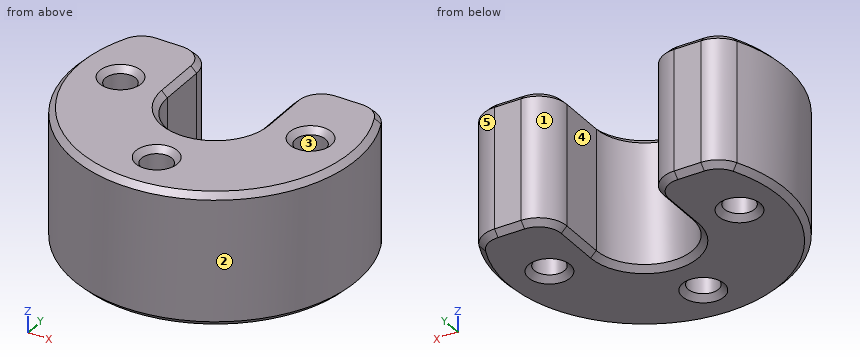
Autodesk Inventor part; units mm, degrees
ref_plane "YZ Plane" through (0, 0, 0) normal (1, 0, 0) x (0, 1, 0)
ref_plane "XZ Plane" through (0, 0, 0) normal (0, 1, 0) x (-1, 0, 0)
ref_plane "XY Plane" through (0, 0, 0) normal (0, 0, 1) x (1, 0, 0)
sketch "Эскиз1" plane through (0, 0, 0) normal (0, 0, 1) x (1, 0, 0)
  circle A0 centre (0, 0) radius 5.1
  circle A1 centre (0, 0) radius 15
  line L0 (0, -21) -> (0, 21) construction
  line L1 (-21, 0) -> (21, 0) construction
  circle A2 centre (0, 0) radius 10.05 construction
  circle A3 centre (-10.05, 0) radius 1.6
  circle A4 centre (0, -10.05) radius 1.6
  circle A5 centre (10.05, 0) radius 1.6
  line L2 (-12.6886, 8) -> (12.6886, 8)
  line L3 (-5.1, 0) -> (-5.1, 8)
  line L4 (5.1, 0) -> (5.1, 8)
  dimension "d0" = 10.2
  dimension "d1" = 30
  dimension "d2" = 20.1
  dimension "d3" = 3.2
  dimension "d4" = 8
extrude "Выдавливание1" add sketch "Эскиз1" along normal blind 14 contours L4 L2 A1 L3 A0
fillet "Сопряжение1" radius 3 4 edges at (-12.6886, 8, 7) (-5.1, 8, 7) (5.1, 8, 7) (12.6886, 8, 7)
chamfer "Фаска1" distance 0.6 angle 45 26 edges at (-5.9787, 7.1213, 14) (-5.1, 2.5, 14) (0, -5.1, 14) (5.1, 2.5, 14) (5.9787, 7.1213, 14) (9.5044, 8, 14) (12.5289, 7.5249, 14) (0, -15, 14) (-12.5289, 7.5249, 14) (-9.5044, 8, 14) (-11.65, 0, 14) (-1.6, -10.05, 14) (8.45, 0, 14) (0, -5.1, 0) (-5.1, 2.5, 0) (-5.9787, 7.1213, 0) (-9.5044, 8, 0) (-12.5289, 7.5249, 0) (0, -15, 0) (12.5289, 7.5249, 0) (9.5044, 8, 0) (5.9787, 7.1213, 0) (5.1, 2.5, 0) (-11.65, 0, 0) (-1.6, -10.05, 0) (8.45, 0, 0)
equation "\"d2\" = 0.5 * d0 + 0.5 * d1"
properties part number "Проставка катушки правая"
Read the model definition and answer for the solid it produces. Units are mm, in the model's axes. Face numbers are marked on the shaded views. A direction names the side the tool comes from. Round coordinates to 2 decimals unless told otherwise and drop trailing zeros. Write each loop counter-clockwise with the first axis right and the second up, starting at its lowest first coordinate (ties: lowest second). Pieces come first, ordered by that corner, then holes.
1. The part is cut by section B-B, the plane z = 5. Determine the outline of the cut face in (x, y), then the cut area to 3 significant figures.
2. Straight lines are drawn through the part: L1, parallel to Y at x = 0, z = 6.25; L2, parallel to Y at x = 9.5, z = 11.25; L3, parallel to X at y = 2.75, z = 6.5. For each, find the intervals that lie inside material, in ascending order.
3. Which of the six approach directions +Z, -Z, +X, -X, +Y, -Y give full straight-line access (tool end or side, diameter ignored) to the marked faces 1 and 2?
4. Determine the mould class of the marked faces 3, 4 and 5 for opening direction Y: pulls with the +Y half, pulls with the -Y half, needs draft (parallel to the pull), parting line crosses it, or undercut.
5. Given pin 1 Ø3.5 at (x, y) = (10.05, 0) entering from -Z; pin 2 Ø1.5 at (y, z) = (2, 10) entering from +X; pin 3 Ø3 at (x, z) = (-6, 9.5) entering from +Y, each flat-ended and moving along its own axis, determine where each tip first touches the part or whether it passes through.
6. The part is cut by section A-A, the plane x = 0. Determine the outline of the cut face in (y, z), then the cut area to 3 significant figures.
Values:
1. outline: (-13.64, 6.25) arc R15 ccw (long way) to (13.64, 6.25) arc R3 ccw to (10.91, 8) - (8.1, 8) arc R3 ccw to (5.1, 5) - (5.1, 0) arc R5.1 cw to (-5.1, 0) - (-5.1, 5) arc R3 ccw to (-8.1, 8) - (-10.91, 8) arc R3 ccw to start; hole circle Ø3.2 at (-10.05, 0); hole circle Ø3.2 at (0, -10.05); hole circle Ø3.2 at (10.05, 0)
1. area: 430 mm2
2. L1: y = -15 to -11.65, -8.45 to -5.1
2. L2: y = -11.61 to -1.5, 1.5 to 8
2. L3: x = -14.75 to -5.1, 5.1 to 14.75
3. face 1: +Z, -Z, +Y
3. face 2: +Z, -Z
4. face 3: undercut
4. face 4: needs draft
4. face 5: pulls with the +Y half
5. pin 1: stops at z = 0.45
5. pin 2: stops at x = 14.95
5. pin 3: stops at y = 7.94
6. outline: (-15, 0.6) - (-14.4, 0) - (-12.25, 0) - (-11.65, 0.6) - (-11.65, 13.4) - (-12.25, 14) - (-14.4, 14) - (-15, 13.4) - close; (-8.45, 0.6) - (-7.85, 0) - (-5.7, 0) - (-5.1, 0.6) - (-5.1, 13.4) - (-5.7, 14) - (-7.85, 14) - (-8.45, 13.4) - close
6. area: 92.4 mm2
